Answer from the drawing. Dimensions are ordinates in mm from the lowest x, y and z of the part. A direction names the side the tool comes from. Round coordinates to 2 decimals unless told otherwise and drop trailing zeros. Loops run counter-clockwise (first coordinate to the right, second up) from the corner with the lowest first, then second, coordinate; pieces in that order, holes last. Notation, with made-up numbers: M 83,22 L 132,22 A19 cw 132,59 Z; hole C 32,-12 d11. An arc over 180 degrees is marked long. Answer as CSV lines item,"result".
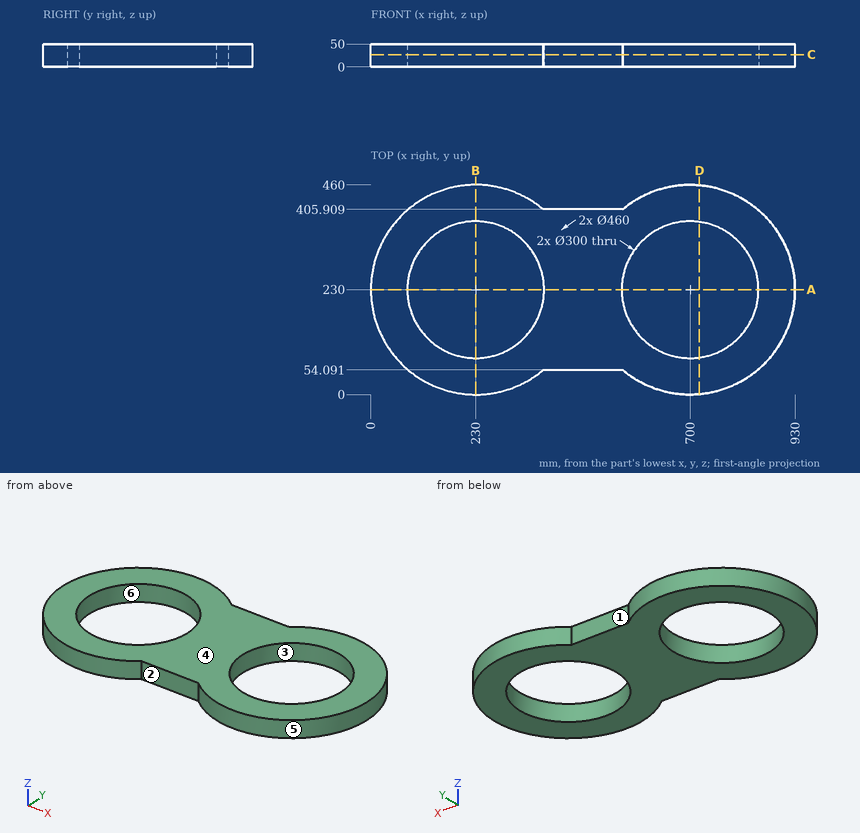
1) Find section A-A, the plane y = 230. Give the vertices of the cut face in (x, z).
Evaluation:
outline,"M 0,0 L 80,0 L 80,50 L 0,50 Z; M 380,0 L 550,0 L 550,50 L 380,50 Z; M 850,0 L 930,0 L 930,50 L 850,50 Z"
2) Find section D-D, the plane x = 720.5. Give the vertices of the cut face in (y, z), then the cut area to 3 significant figures.
Evaluation:
outline,"M 0.92,0 L 81.41,0 L 81.41,50 L 0.92,50 Z; M 378.59,0 L 459.08,0 L 459.08,50 L 378.59,50 Z"
area,"8,050 mm^2"
3) Each of these flat-tipped pins is pushed along its axis until it touches: P1, Ø12, axis at y = 402.5, z = 40, coming from the +X side (1 decimal); P2, Ø1.5, axis at x = 151.5, z = 33.5, coming from the +Y side; P3, Ø5, axis at x = 317.5, z = 24.5, coming from the +Y side. Where does it stop, or does it pass through?
Evaluation:
P1,"stops at x = 858.7"
P2,"stops at y = 446.46"
P3,"stops at y = 443.72"
4) Find section B-B, the plane x = 230. Give the vertices of the cut face in (y, z), then the cut area to 3 significant figures.
Evaluation:
outline,"M 0,0 L 80,0 L 80,50 L 0,50 Z; M 380,0 L 460,0 L 460,50 L 380,50 Z"
area,"8,000 mm^2"
5) Determine the mould class of the marked faces 4, 5 and 6 for opening direction Y: released by +Y, released by -Y, zero draft, split by the parting line, or undercut.
Evaluation:
face 4,"zero draft"
face 5,"split by the parting line"
face 6,"undercut"
6) A tool of negligible diameter and unlimited length cuts with its end or side. For the marked faces 1, 2 and 3, from which of +Z, -Z, +X, -X, +Y, -Y can it reach the whole face along a straight path? Write none if from no direction.
Evaluation:
face 1,"+Z, -Z, +Y"
face 2,"+Z, -Z, -Y"
face 3,"+Z, -Z"
7) Straight lines are drawn through the part: line 1 (X direction, y = 235.5, z = 37.5); line 2 (Y direction, x = 230, z = 34); line 3 (X direction, y = 120, z = 16). For each, find the intervals that lie inside material, in ascending order.
Evaluation:
line 1,"x = 0.07 to 80.1, 379.9 to 550.1, 849.9 to 929.93"
line 2,"y = 0 to 80, 380 to 460"
line 3,"x = 28.01 to 128.02, 331.98 to 598.02, 801.98 to 901.99"
8) Find section C-C, the plane z = 26.5. Give the vertices of the cut face in (x, y).
Evaluation:
outline,"M 378.18,54.09 L 551.82,54.09 A230 ccw long 551.82,405.91 L 378.18,405.91 A230 ccw long Z; hole C 230,230 d300; hole C 700,230 d300"
